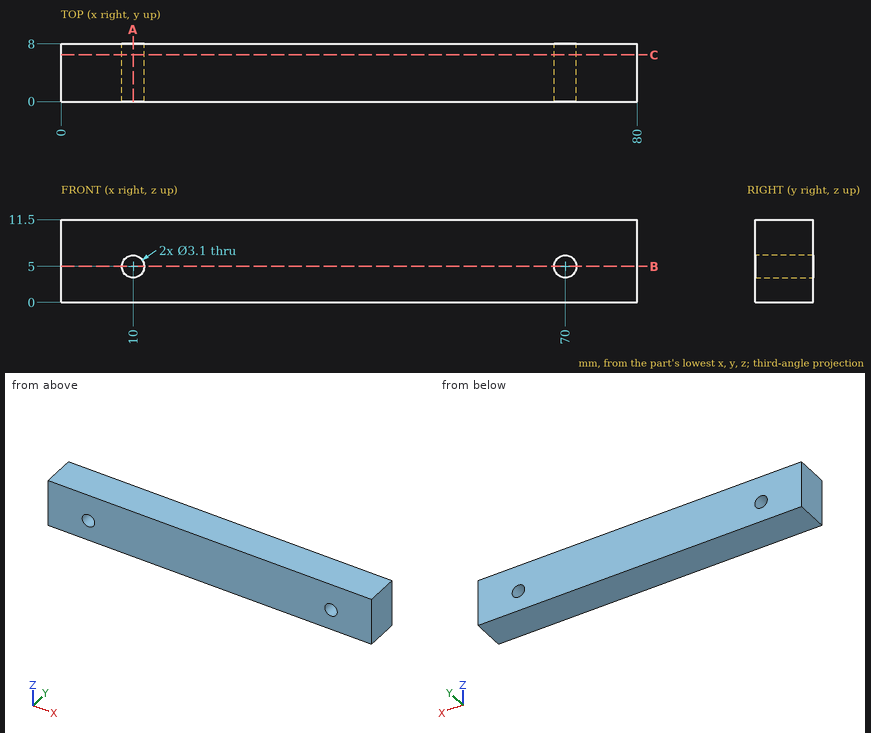
Drawing for the job (mm, zero at the part's lowest x, y, z). Give positions to 0.01 mm unless a question says otherwise; leave off trailing zeros. Write each loop counter-clockwise with the first axis right and the second up, starting at its lowest first coordinate (ties: lowest second). Pieces come first, ordered by that corner, then holes. Notation, with made-up numbers: M -19.5,43 L -13.5,43 A21 cw -13.5,77 Z; hole C 7,-35 d7. An arc over 180 degrees is marked long. Return JSON: item names as keys, results as strings. Group by question number.
(1) Band-saw the part on A-A (x = 10). Give the cut face in (y, z).
(2) Band-saw the part on C-C (y = 6.5). Give the cut face in (x, z).
(3) Drill centre lines: L1, parallel to X at y = 5.25, z = 5; L2, parallel to Z at x = 70, y = 4.5; L3, parallel to X at y = 4, z = 6.25. Where is each one in solid material? Low to high. Write a range as [from, to].
(4) Flat gauge pin, fed straight in: pin 1 Ø1.9 at (x, z) = (10, 5) entering from +Y. Where does the tip first touch, or does it go through?
(5) Band-saw the part on B-B (z = 5). Give the cut face in (x, y), and give its area (3 significant figures).
Entries:
{
 "1": {"outline": "M 0,0 L 8,0 L 8,3.45 L 0,3.45 Z; M 0,6.55 L 8,6.55 L 8,11.5 L 0,11.5 Z"},
 "2": {"outline": "M 0,0 L 80,0 L 80,11.5 L 0,11.5 Z; hole C 10,5 d3.1; hole C 70,5 d3.1"},
 "3": {"L1": "x = [0, 8.45], [11.55, 68.45], [71.55, 80]", "L2": "z = [0, 3.45], [6.55, 11.5]", "L3": "x = [0, 9.08], [10.92, 69.08], [70.92, 80]"},
 "4": {"pin 1": "passes through"},
 "5": {"outline": "M 0,0 L 8.45,0 L 8.45,8 L 0,8 Z; M 11.55,0 L 68.45,0 L 68.45,8 L 11.55,8 Z; M 71.55,0 L 80,0 L 80,8 L 71.55,8 Z", "area": "590 mm^2"}
}
